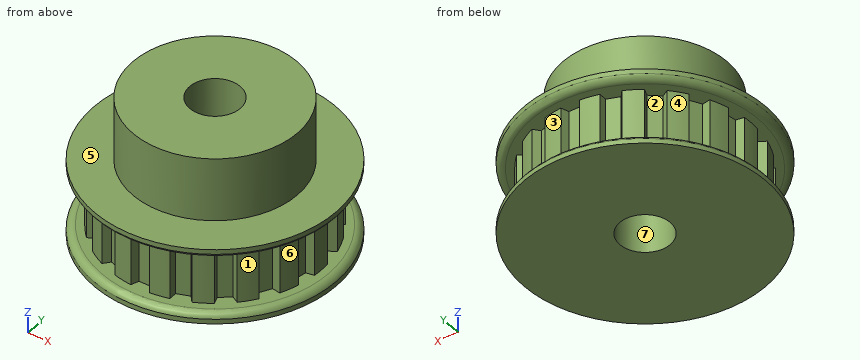
```python
from build123d import *

# Parameters (mm, degrees)
CUT_EXTRUDE1_START = -0.7874
CUT_EXTRUDE1_DEPTH = 14.3002
CIRPATTERN1_COUNT  = 18


with BuildPart() as part:
    # Sketch2 → Revolve1 (revolve)
    with BuildSketch(Plane(origin=(0, 0, 0), x_dir=(0, 0, -1), z_dir=(1, 0, 0)), mode=Mode.PRIVATE) as revolve1_sk:
        with BuildLine():
            Line((-17.4625, 6.35), (17.4625, 6.35))
            Line((17.4625, 6.35), (17.4625, 30.3657))
            Line((17.4625, 30.3657), (16.27505, 30.3657))
            ThreePointArc((16.27505, 30.3657), (15.408910445, 29.58682048), (15.0876, 28.467172932))
            Line((15.0876, 28.467172932), (15.0876, 26.568645864))
            Line((15.0876, 26.568645864), (0.7874, 26.568645864))
            Line((0.7874, 26.568645864), (0.7874, 28.467172932))
            ThreePointArc((0.7874, 28.467172932), (0.466089555, 29.58682048), (-0.40005, 30.3657))
            Line((-0.40005, 30.3657), (-1.5875, 30.3657))
            Line((-1.5875, 30.3657), (-1.5875, 20.6375))
            Line((-1.5875, 20.6375), (-17.4625, 20.6375))
            Line((-17.4625, 20.6375), (-17.4625, 6.35))
        make_face()
    revolve(revolve1_sk.sketch.rotate(Axis((0, 0, 17.4625), (0, 0, -1)), 90), axis=Axis((0, 0, 17.4625), (0, 0, -1)))

    # Sketch3 → Cut-Extrude1 (cut)
    with BuildSketch(Plane.XY.offset(CUT_EXTRUDE1_START)):
        with BuildLine():
            Line((-1.630736704, 24.5618), (1.630736704, 24.5618))
            Line((1.630736704, 24.5618), (2.3241, 26.4668))
            ThreePointArc((2.3241, 26.4668), (0, 26.568645864), (-2.3241, 26.4668))
            Line((-2.3241, 26.4668), (-1.630736704, 24.5618))
        make_face()
    cut_extrude1 = extrude(amount=-CUT_EXTRUDE1_DEPTH, mode=Mode.SUBTRACT)

    # CirPattern1: Cut-Extrude1 ×18 about axis
    cirpattern1_axis = Axis((0, 0, 0), (0, 0, 1))
    for i in range(1, CIRPATTERN1_COUNT):
        add(cut_extrude1.rotate(cirpattern1_axis, i * 360 / CIRPATTERN1_COUNT), mode=Mode.SUBTRACT)


solid = part.part
```
Work out the finished part from the listing and answer in its coordinate system (mm). Face numbers are marked on the shaded views. A direction names the side the tool comes from. Give positions to 0.01 mm unless a question says otherwise; leave off trailing zeros. Order: outer loops, then holes, each group sorted by start corner. A loop starts at its lowest first (then second) coordinate and runs counter-clockwise, first axis right, second up. Notation, with made-up numbers: (21.25, 68.25) -> (40.25, 68.25) arc R10 cw to (40.25, 77.25) -> close; hole circle Ø5 at (-37.75, -5.75). An arc over 180 degrees is marked (long way). Answer as CSV lines item,"result". Start each with the question number.
(1) Section B-B, the plane x = 0 is taken. Write down the section's boundary in (y, z).
(2) Each of these flat-tipped pins is pushed along its axis until it touches: pin 1 Ø1.6 at (y, z) = (24, -6) entering from +X; pin 2 Ø2 at (x, z) = (7.5, -6) entering from +Y; pin 3 Ø4 at (y, z) = (-3.5, 9) entering from -X; pin 4 Ø20.5 at (x, y) = (0, 0) entering from -Z. Where does it stop, or does it pass through?
(3) Consider line 1 along Z through (x, y) = (-16, 21.5); line 2 along Y through (x, z) = (0, -7); line 3 along Y through (x, z) = (0, 9). Determine where each line is inside the solid, lowest interval first.
(4) Section A-A, the plane y = 0 is taken. Write down the section's boundary in (x, z).
(5) Which of the six approach directions +Z, -Z, +X, -X, +Y, -Y give full straight-line access (tool end or side, diameter ignored) to the marked faces 1, 2, 3 and 4?
(6) For a pull along Y with two mould halves and no side action, classify the marked faces 5, 6 and 7 as released by +Y, released by -Y, zero draft, split by the parting line, or undercut.
Entries:
1,outline,"(-30.37, -17.46) -> (-6.35, -17.46) -> (-6.35, 17.46) -> (-20.64, 17.46) -> (-20.64, 1.59) -> (-30.37, 1.59) -> (-30.37, 0.4) arc R2.11 ccw to (-28.47, -0.79) -> (-24.56, -0.79) -> (-24.56, -15.09) -> (-28.47, -15.09) arc R2.11 ccw to (-30.37, -16.28) -> close; (6.35, -17.46) -> (30.37, -17.46) -> (30.37, -16.28) arc R2.11 ccw to (28.47, -15.09) -> (24.56, -15.09) -> (24.56, -0.79) -> (28.47, -0.79) arc R2.11 ccw to (30.37, 0.4) -> (30.37, 1.59) -> (20.64, 1.59) -> (20.64, 17.46) -> (6.35, 17.46) -> close"
2,pin 1,"x = 12.95"
2,pin 2,"y = 25.76"
2,pin 3,"x = -20.58"
2,pin 4,"z = -17.46"
3,line 1,"-17.46 to -15.09, -0.79 to 1.59"
3,line 2,"-24.56 to -6.35, 6.35 to 24.56"
3,line 3,"-20.64 to -6.35, 6.35 to 20.64"
4,outline,"(-30.37, -17.46) -> (-6.35, -17.46) -> (-6.35, 17.46) -> (-20.64, 17.46) -> (-20.64, 1.59) -> (-30.37, 1.59) -> (-30.37, 0.4) arc R2.11 ccw to (-28.47, -0.79) -> (-26.57, -0.79) -> (-26.57, -15.09) -> (-28.47, -15.09) arc R2.11 ccw to (-30.37, -16.28) -> close; (6.35, -17.46) -> (30.37, -17.46) -> (30.37, -16.28) arc R2.11 ccw to (28.47, -15.09) -> (26.57, -15.09) -> (26.57, -0.79) -> (28.47, -0.79) arc R2.11 ccw to (30.37, 0.4) -> (30.37, 1.59) -> (20.64, 1.59) -> (20.64, 17.46) -> (6.35, 17.46) -> close"
5,face 1,"+X, -Y"
5,face 2,"none"
5,face 3,"+X, +Y"
5,face 4,"-X, +Y"
6,face 5,"zero draft"
6,face 6,"released by -Y"
6,face 7,"undercut"
